Check sheet for the modelled part. Datum: model origin and axes. Units: mm. A direction names the side the tool comes from. Round coordinates to 2 decimals unless told otherwise and drop trailing zeros. Order: outer loops, then holes, each group sorted by start corner. A loop starts at its lowest first (then second) coordinate and runs counter-clockwise, first axis right, second up.
```python
from build123d import *

# Parameters (mm, degrees)
F1_W     = 2.92
F1_H     = 15
F1_W_2   = 15
F1_H_2   = 2.92
F2_DEPTH = 2.92


with BuildPart() as f2:
    # F1 (on Front) → F2 (new body)
    with BuildSketch(Plane.XZ):
        with BuildLine():
            Line((0, 55), (0, 0))
            Line((0, 0), (10, 0))
            Line((10, 0), (10, 48))
            ThreePointArc((10, 48), (10.5857864376, 49.4142135624), (12, 50))
            Line((12, 50), (37, 50))
            ThreePointArc((37, 50), (38.4142135624, 49.4142135624), (39, 48))
            Line((39, 48), (39, -19.8143487114))
            Line((39, -19.8143487114), (61.7363576694, -19.8143487114))
            Line((61.7363576694, -19.8143487114), (174.84, 29.0905267951))
            Line((174.84, 29.0905267951), (174.84, 55))
            ThreePointArc((174.84, 55), (173.3755339059, 58.5355339059), (169.84, 60))
            Line((169.84, 60), (5, 60))
            ThreePointArc((5, 60), (1.4644660941, 58.5355339059), (0, 55))
        make_face()
        with Locations((45.46, -7.5)):
            Rectangle(F1_W, F1_H, mode=Mode.SUBTRACT)
        with Locations((5, 17.5)):
            Rectangle(F1_W, F1_H, mode=Mode.SUBTRACT)
        with Locations((84.42, 40)):
            Rectangle(F1_W_2, F1_H_2, mode=Mode.SUBTRACT)
        with Locations((24.5, 55)):
            Rectangle(F1_W_2, F1_H_2, mode=Mode.SUBTRACT)
        with Locations((45.46, 42.5)):
            Rectangle(F1_W, F1_H, mode=Mode.SUBTRACT)
        with Locations((129.42, 40)):
            Rectangle(F1_W_2, F1_H_2, mode=Mode.SUBTRACT)
        with Locations((168.38, 42.5)):
            Rectangle(F1_W, F1_H, mode=Mode.SUBTRACT)
    extrude(amount=F2_DEPTH)


solid = f2.part
```
Item 1: Scan lines: line 1 along Z through (x, y) = (45.5, -2.45); line 2 along Z through (x, y) = (31, -1.4); line 3 along X through (y, z) = (-1.7, 48). Record each from-to range of solid material in increasing order.
Answer:
line 1: z = -19.81 to -15, 0 to 35, 50 to 60
line 2: z = 50 to 53.54, 56.46 to 60
line 3: x = 0 to 10, 39 to 44, 46.92 to 166.92, 169.84 to 174.84
Item 2: Access from +Z, -Z, +X, -X, +Y, -Y to the whole of each face (thin tool, end or side, straight path). Record for faces 4 (the flat face through (86, -2.92, 30)), 5 (the flat face through (44, -1, -8)).
Answer:
face 4: +Z, -Z, +X, -X, -Y
face 5: +Y, -Y
Item 3: Sectioned sample at C-C (z = 6). Record the cut outline in (x, y), and give its area (3 significant figures).
Answer:
outline: (0, -2.92) - (10, -2.92) - (10, 0) - (0, 0) - close; (39, -2.92) - (121.44, -2.92) - (121.44, 0) - (39, 0) - close
area: 270 mm2
Item 4: Go/stop test with flat-tipped pins: P1, Ø1.5, axis at y = -2, z = 46, coming from the -X side; P2, Ø0.9, axis at x = 25.5, y = -1, coming from the -Z side; P3, Ø1.5, axis at y = -1, z = -7.5, coming from the +X side; P4, Ø12, axis at x = 28.5, z = 18.5, coming from the +Y side. Record where each tip stops, or that it passes through.
Answer:
P1: stops at x = 0
P2: stops at z = 50
P3: stops at x = 91.95
P4: passes through
Item 5: Release check for a two-part mould opening along Z. For faces 1 (the flat face through (0, -1, 28)), 2 (the cylindrical face through (173.41, -1.44, 58.5)), 3 (the flat face through (84, -1, 41.46)) record: released by +Z, released by -Z, zero draft, split by the parting line, or undercut.
Answer:
face 1: zero draft
face 2: released by +Z
face 3: undercut
Item 6: Sectioned sample at A-A (z = 46). Record the cut outline in (x, y), and give its area (3 significant figures).
Answer:
outline: (0, -2.92) - (10, -2.92) - (10, 0) - (0, 0) - close; (39, -2.92) - (44, -2.92) - (44, 0) - (39, 0) - close; (46.92, -2.92) - (166.92, -2.92) - (166.92, 0) - (46.92, 0) - close; (169.84, -2.92) - (174.84, -2.92) - (174.84, 0) - (169.84, 0) - close
area: 409 mm2
Item 7: Sectioned sample at D-D (y = -0.5). State how many separate pieces and enclosed holes the cut face has, and give its area (3 significant figures).
Answer:
separate pieces: 1
enclosed holes: 7
area: 8,650 mm2
Item 8: Sectioned sample at B-B (z = 22.5). Record the cut outline in (x, y).
Answer:
outline: (0, -2.92) - (3.54, -2.92) - (3.54, 0) - (0, 0) - close; (6.46, -2.92) - (10, -2.92) - (10, 0) - (6.46, 0) - close; (39, -2.92) - (159.6, -2.92) - (159.6, 0) - (39, 0) - close
